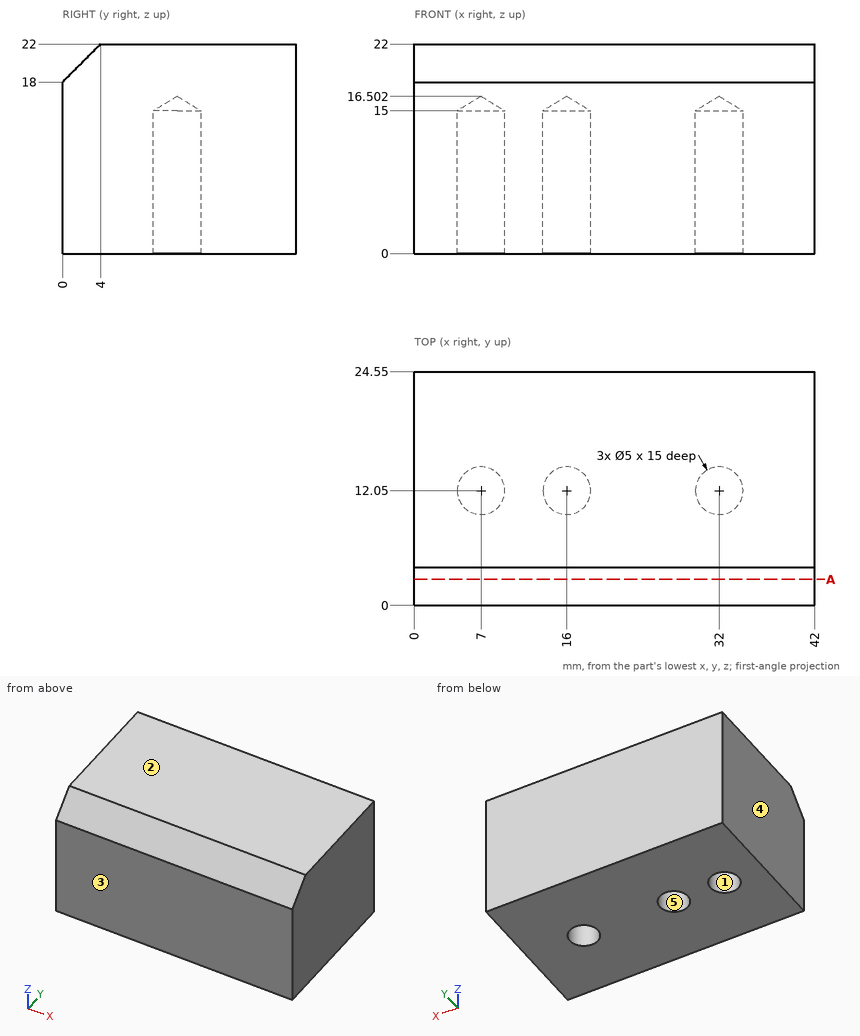
Can you work these out from the drawing? Everything is in mm from the part's minimum corner. A direction names the side the tool comes from. Give positions to 0.01 mm unless a question says otherwise; leave off trailing zeros. Write each loop counter-clockwise with the first axis right and the second up, starting at its lowest first coordinate (ties: lowest second). Pieces come first, ordered by that corner, then holes. Notation, with made-up numbers: (55, -28) -> (86, -28) arc R16 cw to (86, -4) -> close; hole circle Ø9 at (-0.5, -14.75). An arc over 180 degrees is marked (long way). Write each question's results on one line, items separated by ' | '.
Item 1: On a 3-axis mill with a long thin cutter (end or side, diameter ignored), from which of +Z, -Z, +X, -X, +Y, -Y can I reach the whole of each face in a straight line? I mean the marked faces 4 and 5. Say none if no direction works.
Output:
face 4: +Z, -Z, -X, +Y, -Y | face 5: -Z
Item 2: We'd pull the mould along Y, two halves only. Please class the marked faces 1, 2 and 3: pulls with the +Y half, pulls with the -Y half, needs draft (parallel to the pull), parting line crosses it, or undercut.
Output:
face 1: undercut | face 2: needs draft | face 3: pulls with the -Y half
Item 3: If I drill on L1, parallel to Y at x = 32, z = 5.75; L2, parallel to X at y = 13.25, z = 4.25; L3, parallel to Y at x = 30, z = 4.75, over which ranges is the centre line in solid material (lowest first)?
Output:
L1: y = 0 to 9.55, 14.55 to 24.55 | L2: x = 0 to 4.81, 9.19 to 13.81, 18.19 to 29.81, 34.19 to 42 | L3: y = 0 to 10.55, 13.55 to 24.55
Item 4: Suppose I cut it at A-A on y = 2.75. Write out the boundary of the cut face in (x, z), plus the area to 4 significant figures.
Output:
outline: (0, 0) -> (42, 0) -> (42, 20.75) -> (0, 20.75) -> close | area: 871.5 mm^2
Item 5: For pin 1 Ø4 at (x, y) = (7, 12.05) entering from -Z, with a flat end and sliding along its axis, tell me the tip position at first contact or that it passes through.
Output:
pin 1: stops at z = 15.3
